Geometry check sheet. Reference: drawing and pictorial views, mm from the part's lowest x, y, z. Give positions to 0.01 mm unless a question says otherwise; leave off trailing zeros. Order: outer loops, then holes, each group sorted by start corner. A loop starts at its lowest first (then second) coordinate and runs counter-clockwise, first axis right, second up.
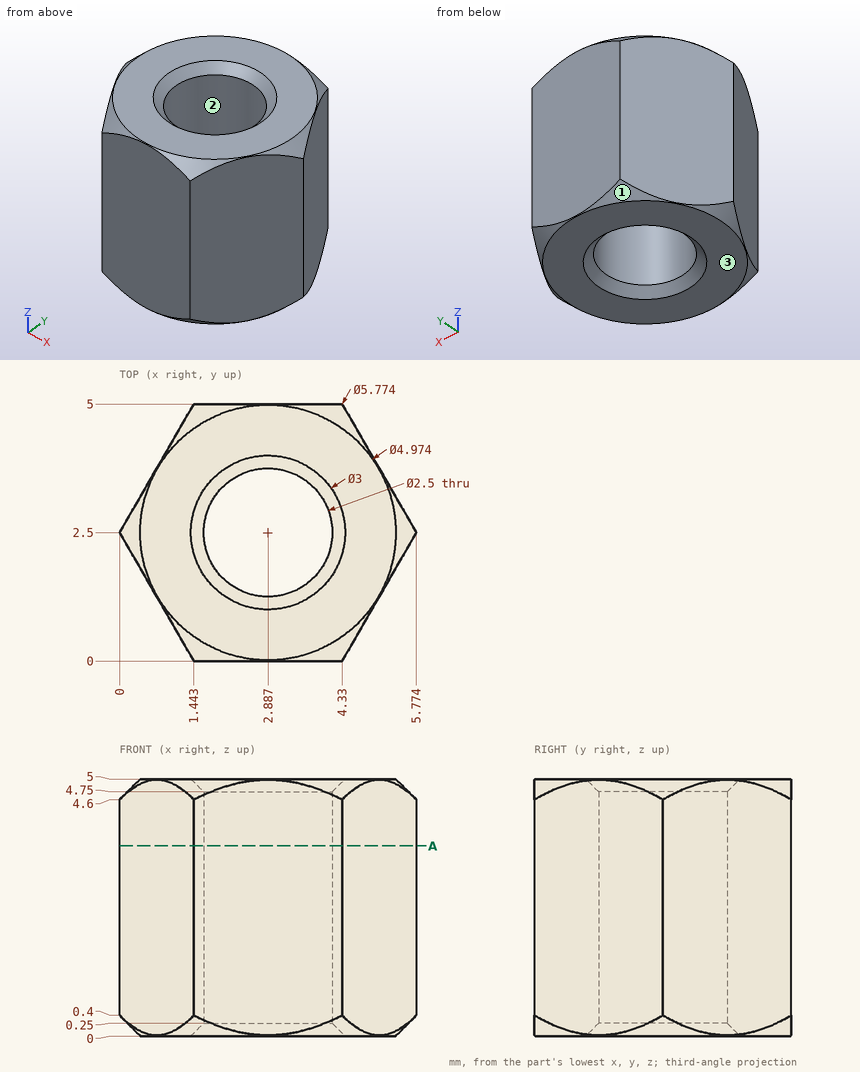
1) Material ranges on L1, parallel to Y at x = 2.55, z = 3.1 (1 decimal); L2, parallel to Y at x = 2.2, z = 3.9 (1 decimal); L3, parallel to X at y = 2.9, z = 1.35, recorded low to high.
Recorded:
L1: y = 0 to 1.3, 3.7 to 5
L2: y = 0 to 1.5, 3.5 to 5
L3: x = 0.23 to 1.7, 4.07 to 5.54
2) Section check A-A, the plane z = 3.7. Record the cut outline in (x, y).
Recorded:
outline: (0, 2.5) - (1.44, 0) - (4.33, 0) - (5.77, 2.5) - (4.33, 5) - (1.44, 5) - close; hole circle Ø2.5 at (2.89, 2.5)
3) Depth check by flat-ended pin: pin 1 Ø1 at (y, z) = (3.5, 0.5) entering from +X (1 decimal). Enter the tip coordinate at first touch or a pass-through.
Recorded:
pin 1: stops at x = 5.5
4) Draft check along X on the marked faces 1, 2 and 3. Enter one of: +X half, -X half, draft (parallel to the pull), parting line (faces both ways), or undercut.
Recorded:
face 1: parting line
face 2: undercut
face 3: draft
